Autodesk Inventor part; units mm, degrees
ref_plane "YZ Plane" through (0, 0, 0) normal (1, 0, 0) x (0, 1, 0)
ref_plane "XZ Plane" through (0, 0, 0) normal (0, 1, 0) x (-1, 0, 0)
ref_plane "XY Plane" through (0, 0, 0) normal (0, 0, 1) x (1, 0, 0)
sketch "Skizze3" plane through (0, 0, 0) normal (0, 1, 0) x (-1, 0, 0)
  line L0 (0, 0) -> (0, -70)
  line L1 (0, -70) -> (35, -70)
  line L2 (35, -70) -> (35, 0)
  line L3 (35, 0) -> (0, 0)
  point P0 (30, -25)
  point P1 (30, -45)
  point P2 (35, -35)
  point P3 (10, -15)
  point P4 (10, -55)
  dimension "d4" = 35
  dimension "d5" = 70
  dimension "d6" = 5
  dimension "d7" = 5
  dimension "d8" = 10
  dimension "d9" = 10
  dimension "d10" = 15
  dimension "d11" = 15
  dimension "d12" = 10
  dimension "d13" = 10
extrude "Extrusion3" add sketch "Skizze3" along normal blind 8
hole "Bohrung1" at (-30, 0, -45) at (-30, 0, -25) direction (0, 1, 0) diameter 5 depth 6
sketch "Skizze4" plane through (0, 8, 0) normal (0, 1, 0) x (1, 0, 0)
  point P0 (0, 0)
  point P1 (-10, 15)
  point P2 (-10, 55)
  point P3 (-10, 15)
  point P4 (-10, 55)
hole "Bohrung2" at (-10, 8, -15) at (-10, 8, -55) direction (0, -1, 0) diameter 5 end through all counterbore diameter 10 counterbore depth 5.4
chamfer "Fase1" distance 2 angle 45 4 edges at (-35, 4, 0) (0, 4, 0) (0, 4, -70) (-35, 4, -70)
properties part number "BT503_trajan20_21" material "Kunststoff, undurchsichtig Schwarz"
Geometry check sheet. Reference: the model listing, model coordinates, mm. A direction names the side the tool comes from. Round coordinates to 2 decimals unless told otherwise and drop trailing zeros. Order: outer loops, then holes, each group sorted by start corner. A loop starts at its lowest first (then second) coordinate and runs counter-clockwise, first axis right, second up. Notation, with made-up numbers: (18.5, -26.5) - (44.5, -26.5) arc R33 cw to (44.5, 11.5) - close; hole circle Ø7 at (-2.75, 89.5). An arc over 180 degrees is marked (long way). Use a Markdown table: item, result. Add a question column.
(1) Sectioned sample at D-D, the plane z = -25. Enter the section's corners in (x, y), and give its area (3 significant figures).
(2) Sectioned sample at A-A, the plane z = -55. Enter the section's corners in (x, y).
(3) Release check for a two-part mould opening along X. For faces 4 (the flat face through (-34, 4, -69)), 5 (the flat face through (0, 4, -35)), 6 (the flat face through (-8, 2.6, -13)) record: pulls with the +X half, pulls with the -X half, needs draft (parallel to the pull), parting line crosses it, or undercut.
(4) Depth check by flat-ended pin: pin 1 (8 mm diameter, centred on x = -30, z = -45, fed in from -Y); pin 2 (4 mm diameter, centred on x = -10, z = -15, fed in from -Y); pin 3 (3 mm diameter, centred on x = -30, z = -25, fed in from -Y). Enter the tip coordinate at first touch or a pass-through.
(5) Sectioned sample at B-B, the plane y = 5. Enter the section's corners in (x, z), and give its area (3 significant figures).
(6) Material ranges on line 1 along Z through (x, y) = (-10, 4.4); line 2 along Z through (x, y) = (-30, 1.45); line 3 along X through (y, z) = (2.1, -55), recorded low to high. Write a range as [from, to].
(7) Tool access check on faces 1 (the cylindrical face through (-31.69, 3.04, -23.16)), 2 (the cylindrical face through (-13, 5, -19)), 3 (the flat face through (-17, 8, -35)). Record the directions out of +Z, -Z, +X, -X, +Y, -Y that give a thin tool (end or side, any length) a straight path to the whole face; none if there is none.
(8) Sectioned sample at C-C, the plane x = -14. Enter the section's corners in (y, z), and give its area (3 significant figures).
Answers below:
| question | item | result |
|---|---|---|
| 1 | outline | (-35, 0) - (-32.5, 0) - (-32.5, 6) - (-27.5, 6) - (-27.5, 0) - (0, 0) - (0, 8) - (-35, 8) - close |
| 1 | area | 250 mm² |
| 2 | outline | (-35, 0) - (-12.5, 0) - (-12.5, 2.6) - (-15, 2.6) - (-15, 8) - (-35, 8) - close; (-7.5, 0) - (0, 0) - (0, 8) - (-5, 8) - (-5, 2.6) - (-7.5, 2.6) - close |
| 3 | face 4 | pulls with the -X half |
| 3 | face 5 | pulls with the +X half |
| 3 | face 6 | undercut |
| 4 | pin 1 | y = 0 |
| 4 | pin 2 | through |
| 4 | pin 3 | y = 6 |
| 5 | outline | (-35, -68) - (-33, -70) - (-2, -70) - (0, -68) - (0, -2) - (-2, 0) - (-33, 0) - (-35, -2) - close; hole circle Ø5 at (-30, -45); hole circle Ø5 at (-30, -25); hole circle Ø10 at (-10, -55); hole circle Ø10 at (-10, -15) |
| 5 | area | 2,250 mm² |
| 6 | line 1 | [-70, -60], [-50, -20], [-10, 0] |
| 6 | line 2 | [-70, -47.5], [-42.5, -27.5], [-22.5, 0] |
| 6 | line 3 | [-35, -12.5], [-7.5, 0] |
| 7 | face 1 | -Y |
| 7 | face 2 | +Y |
| 7 | face 3 | +Z, -Z, +X, -X, +Y |
| 8 | outline | (0, -70) - (8, -70) - (8, -58) - (2.6, -58) - (2.6, -52) - (8, -52) - (8, -18) - (2.6, -18) - (2.6, -12) - (8, -12) - (8, 0) - (0, 0) - close |
| 8 | area | 495 mm² |
